Could you check a few things on this model? Use its own coordinates, in mm. Face numbers are marked on the shaded views. A direction names the side the tool comes from. Round coordinates to 2 decimals unless told otherwise and drop trailing zeros. Write each loop counter-clockwise with the first axis right and the second up, starting at its lowest first coordinate (ties: lowest second). Pieces come first, ordered by that corner, then holes. Notation, with made-up numbers: (-1, -3.5) -> (40, -3.5) arc R29 ccw to (40, 32.5) -> close; hole circle Ø9 at (26, -15.75). An arc over 180 degrees is marked (long way). Answer in a Markdown table with one row per item. Add a question column.
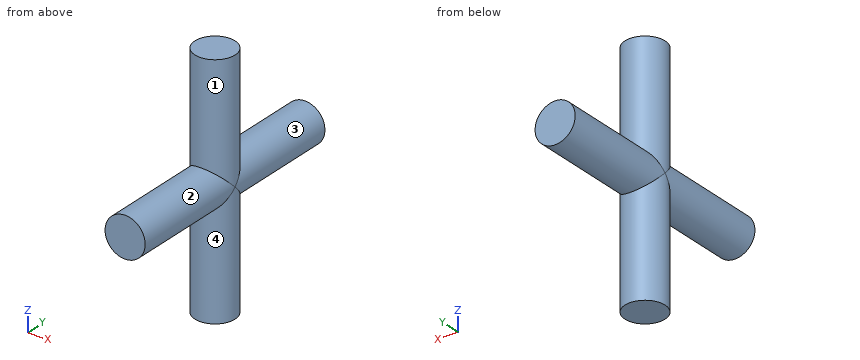
```python
from build123d import *

# Parameters (mm, degrees)
SKETCH1_W                = 1.016
SKETCH1_H                = 6.096
BOSS_EXTRUDE1_DEPTH      = 6.096
BOSS_EXTRUDE1_DEPTH_BACK = 6.096
SKETCH2_R                = 1.016
BOSS_EXTRUDE2_START      = 6.096
SKETCH3_R                = 1.016
BOSS_EXTRUDE2_DEPTH      = 6.096


with BuildPart() as part:
    # Sketch1 → Revolve2 (revolve)
    with BuildSketch(Plane(origin=(0, 0, 0), x_dir=(1, 0, 0), z_dir=(0, 1, 0)), mode=Mode.PRIVATE) as revolve2_sk:
        with Locations((-0.508, 3.048)):
            Rectangle(SKETCH1_W, SKETCH1_H)
    revolve(revolve2_sk.sketch.rotate(Axis((0, 0, 0), (0, 0, -1)), 180), axis=Axis((0, 0, 0), (0, 0, -1)))

    # Sketch2 → Boss-Extrude1 (add, two sides: drawn at the far end of the back side and taken through both)
    with BuildSketch(Plane(origin=(0, 0, 0), x_dir=(1, 0, 0), z_dir=(0, 1, 0)).offset(-BOSS_EXTRUDE1_DEPTH_BACK)):
        with Locations(Location((0, 0, 0), (0, 0, 270))):
            Circle(SKETCH2_R)
    extrude(amount=BOSS_EXTRUDE1_DEPTH + BOSS_EXTRUDE1_DEPTH_BACK)

    # Sketch3 → Boss-Extrude2 (add)
    with BuildSketch(Plane.XY.offset(BOSS_EXTRUDE2_START)):
        Circle(SKETCH3_R)
    extrude(amount=-BOSS_EXTRUDE2_DEPTH)


solid = part.part
```
(1) Suppose I cut it at A-A, the plane x = 0. Please give me the cut outline in (y, z), then the cut area to 3 significant figures.
(2) Suppose I cut it at D-D, the plane x = 0.7. Please give me the cut outline in (y, z), then the cut area to 3 significant figures.
(3) Suppose I cut it at B-B, the plane z = 2.75. Please give me the cut outline in (x, y), then the cut area to 3 significant figures.
(4) I need wall thicknesses on L1, parallel to Y at x = -0.05, z = 1.25; L2, parallel to Z at x = -0.3, y = -4.75; L3, parallel to Z at x = 0.75, y = -1.5. Which ranges of each line are inside material? Lowest first, please.
(5) Suppose I cut it at C-C, the plane y = 0.5. Please give me the cut outline in (x, z), then the cut area to 3 significant figures.
(6) On a 3-axis mill with a long thin cutter (end or side, diameter ignored), from which of +Z, -Z, +X, -X, +Y, -Y can I reach the whole of each face in a straight line? I mean the marked faces 1, 2, 3 and 4. Say none if no direction works.
(7) For P1, Ø1, axis at x = 0.5, z = -4.5, coming from the +Y side, with a flat end and sliding along its axis, tell me the tip position at first contact or that it passes through.
Response:
| question | item | result |
|---|---|---|
| 1 | outline | (-6.1, -1.02) -> (-1.02, -1.02) -> (-1.02, -6.1) -> (1.02, -6.1) -> (1.02, -1.02) -> (6.1, -1.02) -> (6.1, 1.02) -> (1.02, 1.02) -> (1.02, 6.1) -> (-1.02, 6.1) -> (-1.02, 1.02) -> (-6.1, 1.02) -> close |
| 1 | area | 45.4 mm² |
| 2 | outline | (-6.1, -0.74) -> (-0.74, -0.74) -> (-0.74, -6.1) -> (0.74, -6.1) -> (0.74, -0.74) -> (6.1, -0.74) -> (6.1, 0.74) -> (0.74, 0.74) -> (0.74, 6.1) -> (-0.74, 6.1) -> (-0.74, 0.74) -> (-6.1, 0.74) -> close |
| 2 | area | 33.7 mm² |
| 3 | outline | circle Ø2.03 at (0, 0) |
| 3 | area | 3.24 mm² |
| 4 | L1 | -1.01 to 1.01 |
| 4 | L2 | -0.97 to 0.97 |
| 4 | L3 | -0.69 to 0.69 |
| 5 | outline | (-0.88, -6.1) -> (0.88, -6.1) -> (0.88, -0.5) arc R1.02 ccw to (0.88, 0.5) -> (0.88, 6.1) -> (-0.88, 6.1) -> (-0.88, 0.5) arc R1.02 ccw to (-0.88, -0.5) -> close |
| 5 | area | 21.7 mm² |
| 6 | face 1 | +Z |
| 6 | face 2 | -Y |
| 6 | face 3 | +Y |
| 6 | face 4 | -Z |
| 7 | P1 | y = 1.02 |
